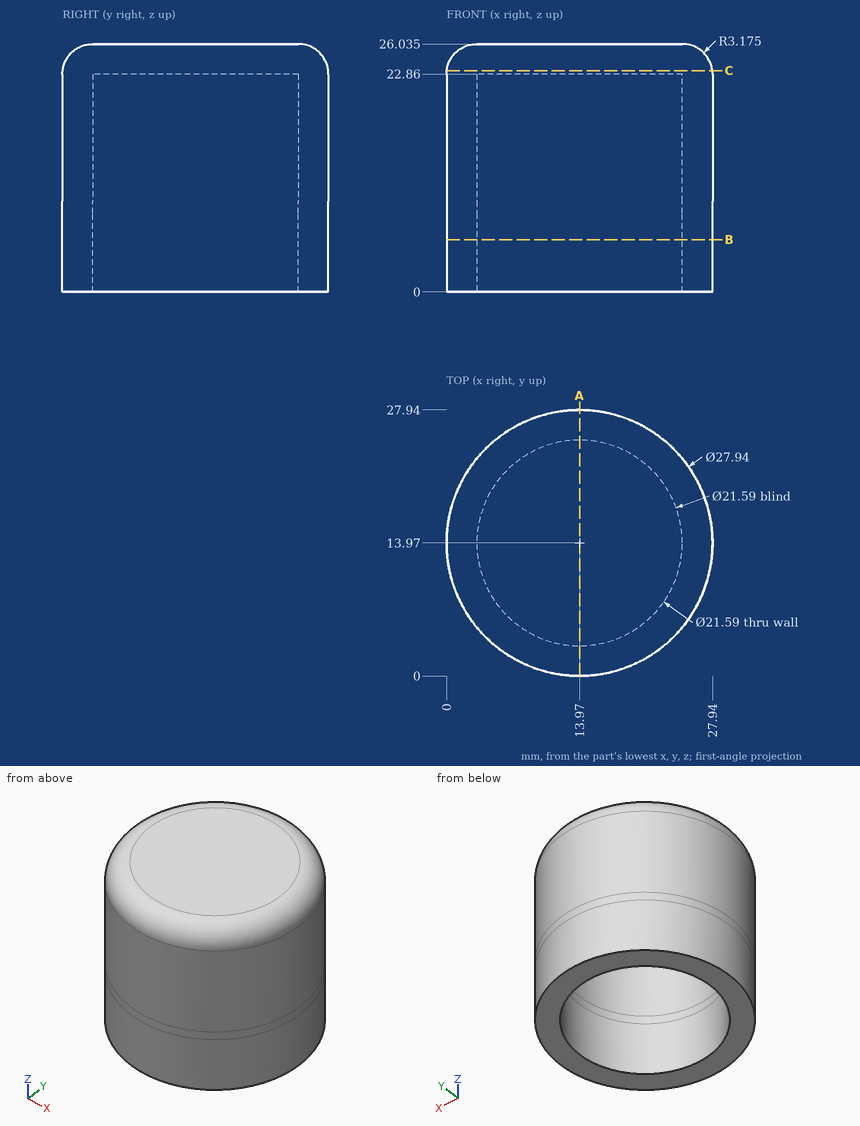
Input: dimensioned drawing with shaded views. Units: mm. Origin: part minimum x, y, z. Round coordinates to 2 decimals unless told otherwise and drop trailing zeros. Order: outer loops, then holes, each group sorted by start corner. A loop starts at its lowest first (then second) coordinate and runs counter-clockwise, first axis right, second up.
Q1. Material intervals for probe 1 along Y at (x, z) = (13.97, 17) (3 decimals); probe 2 along Y at (x, z) = (16, 18); probe 3 along Z at (x, y) = (9.75, 19.75) (3 decimals), sorted ascending.
Result sheet:
probe 1: y = 0 to 3.175, 24.765 to 27.94
probe 2: y = 0.15 to 3.37, 24.57 to 27.79
probe 3: z = 22.86 to 26.035
Q2. Section B-B, the plane z = 5.5. Output: boundary loops of the cut face in (x, y) (3 decimals).
Result sheet:
outline: circle Ø27.94 at (13.97, 13.97); hole circle Ø21.59 at (13.97, 13.97)
Q3. Pin query (flat end, axial travel): pin 1 (6 mm diameter, centred on x = 6.5, y = 13, fed in from -Z); pin 2 (2 mm diameter, centred on x = 7.5, y = 25, fed in from -Z); pin 3 (4 mm diameter, centred on y = 4, z = 16, fed in from +X); pin 4 (6 mm diameter, centred on x = 9.5, z = 7.5, fed in from -Y). Return the tip coordinate at first contact, or that it passes through.
Result sheet:
pin 1: stops at z = 22.86
pin 2: stops at z = 0
pin 3: stops at x = 25.44
pin 4: stops at y = 0.08
Q4. Section A-A, the plane x = 13.97. Output: boundary loops of the cut face in (y, z) (3 decimals).
Result sheet:
outline: (0, 0) - (3.175, 0) - (3.175, 22.86) - (24.765, 22.86) - (24.765, 0) - (27.94, 0) - (27.94, 22.86) arc R3.175 ccw to (24.765, 26.035) - (3.175, 26.035) arc R3.175 ccw to (0, 22.86) - close
Q5. Section C-C, the plane z = 23.25. Output: boundary loops of the cut face in (x, y).
Result sheet:
outline: circle Ø27.89 at (13.97, 13.97)
